```python
from build123d import *

# Parameters (mm, degrees)
SKETCH1_W           = 76
SKETCH1_H           = 56
SKETCH1_R           = 1.5
BOSS_EXTRUDE1_DEPTH = 1.5
FILLET1_R           = 3.5
SKETCH3_W           = 63
SKETCH3_H           = 7.55
BOSS_EXTRUDE3_DEPTH = 10
SKETCH4_W           = 65
SKETCH4_H           = 18.75
BOSS_EXTRUDE4_DEPTH = 15.3


with BuildPart() as part:
    # Sketch1 → Boss-Extrude1 (new body)
    with BuildSketch(Plane(origin=(0, 0, 0), x_dir=(1, 0, 0), z_dir=(0, 1, 0))):
        with Locations((38, -28)):
            Rectangle(SKETCH1_W, SKETCH1_H)
        with Locations(Location((72.8, -52.8, 0), (0, 0, 270))):
            Circle(SKETCH1_R, mode=Mode.SUBTRACT)
        with Locations(Location((72.8, -3.2, 0), (0, 0, 270))):
            Circle(SKETCH1_R, mode=Mode.SUBTRACT)
        with Locations(Location((3.2, -3.2, 0), (0, 0, 270))):
            Circle(SKETCH1_R, mode=Mode.SUBTRACT)
        with Locations(Location((3.2, -52.8, 0), (0, 0, 270))):
            Circle(SKETCH1_R, mode=Mode.SUBTRACT)
    extrude(amount=BOSS_EXTRUDE1_DEPTH)

    # Fillet1
    fillet1_edges = [part.edges().sort_by_distance(p)[0] for p in [
        (0, 0.75, 56),
        (0, 0.75, 0),
        (76, 0.75, 0),
        (76, 0.75, 56),
    ]]
    fillet(fillet1_edges, radius=FILLET1_R)

    # Sketch3 → Boss-Extrude3 (add)
    with BuildSketch(Plane(origin=(0, 1.5, 0), x_dir=(1, 0, 0), z_dir=(0, 1, 0))):
        with Locations((38.5, -48.225)):
            Rectangle(SKETCH3_W, SKETCH3_H)
    extrude(amount=BOSS_EXTRUDE3_DEPTH)

    # Sketch4 → Boss-Extrude4 (add)
    with BuildSketch(Plane(origin=(0, 1.5, 0), x_dir=(1, 0, 0), z_dir=(0, 1, 0))):
        with Locations((38.794123638, -33.130364422)):
            Rectangle(SKETCH4_W, SKETCH4_H)
    extrude(amount=BOSS_EXTRUDE4_DEPTH)


solid = part.part
```
For this review, take the finished solid that the model builds, in its own axes (mm). A direction names the side the tool comes from. Coordinates: 2 decimals unless noted, no trailing zeros. Write each loop counter-clockwise with the first axis right and the second up, starting at its lowest first coordinate (ties: lowest second). Pieces come first, ordered by that corner, then holes.
(1) Wall thickness on probe 1 along Z at (x, y) = (72.8, 1.2); probe 2 along X at (y, z) = (1.1, 3.2); probe 3 along Z at (x, y) = (13.5, 9): over which ranges is each line inside the solid? List them lowest first.
(2) Add section C-C on z = 29. Give the boundary of the cut face in (x, y).
(3) Add section D-D on x = 5.5. Give the boundary of the cut face in (y, z), then the cut area to 3 significant figures.
(4) Tool access review of faces 5 (the face through (38, 9, 42.505)), 6 (the face through (38, 9, 23.755)), 7 (the face through (70, 6, 48)), 8 (the face through (38, 11.5, 48)), 9 (the face through (6.294, 9, 33)): name each direction out of +Z, -Z, +X, -X, +Y, -Y from which nothing blocks a thin tool from reaching the whole face with its end or side.
(5) For pin 1 Ø3 at (x, y) = (59.5, 10.5) entering from -Z; pin 2 Ø8.5 at (x, z) = (41.5, 49.5) entering from +Y; pin 3 Ø4 at (x, z) = (3.2, 3.2) entering from +Y, all flat-tipped, find the tip position at first contact; note any pin that passes through.
(6) Add section A-A on x = 50. Give the boundary of the cut face in (y, z).
(7) Add section B-B on z = 45.5. Give the boundary of the cut face in (x, y), then the cut area to 3 significant figures.
(8) The part is to be moulded in two halves that separate along X. For faces 1 (the face through (38, 1, 0)), 2 (the face through (7, 6, 48)), 3 (the face through (71.294, 9, 33)), 4 (the face through (3.65, 0.74, 54.23)), say which applies: +X half, -X half, draft (parallel to the pull), parting line (faces both ways), or undercut.
Answer sheet:
1. probe 1: z = 0.01 to 1.7, 4.7 to 51.3, 54.3 to 55.99
1. probe 2: x = 0.01 to 1.7, 4.7 to 71.3, 74.3 to 75.99
1. probe 3: z = 23.76 to 42.51, 44.45 to 52
2. outline: (0, 0) - (76, 0) - (76, 1.5) - (71.29, 1.5) - (71.29, 16.8) - (6.29, 16.8) - (6.29, 1.5) - (0, 1.5) - close
3. outline: (0, 0) - (1.5, 0) - (1.5, 56) - (0, 56) - close
3. area: 84.0 mm2
4. face 5: +X, -X, +Y
4. face 6: -Z, +X, -X, +Y
4. face 7: +Z, +X, +Y
4. face 8: +Z, +X, -X, +Y
4. face 9: +Z, -Z, -X, +Y
5. pin 1: stops at z = 23.76
5. pin 2: stops at y = 11.5
5. pin 3: stops at y = 1.5
6. outline: (0, 0) - (1.5, 0) - (1.5, 23.76) - (16.8, 23.76) - (16.8, 42.51) - (1.5, 42.51) - (1.5, 44.45) - (11.5, 44.45) - (11.5, 52) - (1.5, 52) - (1.5, 56) - (0, 56) - close
7. outline: (0, 0) - (76, 0) - (76, 1.5) - (70, 1.5) - (70, 11.5) - (7, 11.5) - (7, 1.5) - (0, 1.5) - close
7. area: 744 mm2
8. face 1: draft
8. face 2: -X half
8. face 3: +X half
8. face 4: undercut
